Check sheet for the modelled part. Datum: model origin and axes. Units: mm. A direction names the side the tool comes from. Round coordinates to 2 decimals unless told otherwise and drop trailing zeros. Order: outer loops, then holes, each group sorted by start corner. A loop starts at its lowest first (then second) coordinate and runs counter-clockwise, first axis right, second up.
Q1. Cross-section at C-C on x = 13. Record the cut outline in (y, z), then the cut area to 3 significant figures.
Q2. Mould release check, pull along Y, two halves, no side actions. Record for faces 5 (the flat face through (2, -2, 0)), 6 (the flat face through (-4, 0, 0)), 7 (the cylindrical face through (13.68, 4.08, -5.65)), 8 (the cylindrical face through (11.631, 5.175, -4.771)): +Y half, -Y half, draft (parallel to the pull), parting line (faces both ways), or undercut.
Q3. Cross-section at D-D on z = 5. Record the cut outline in (x, y).
Q4. Scan lines: probe 1 along Z at (x, y) = (0, 3.5); probe 2 along Y at (x, z) = (9.25, -2.4); probe 3 along Z at (x, y) = (10, 9.5). Record each from-to range of solid material in increasing order.
Q5. Depth check by flat-ended pin: P1, Ø4, axis at x = 3.5, z = 0, coming from the +Y side; P2, Ø5, axis at x = 9.25, y = 7, coming from the +Z side; P3, Ø4, axis at x = -3, z = -4, coming from the +Y side; P4, Ø0.5, axis at x = -4.5, z = -0.5, coming from the +Y side. Enter the tip coordinate at first touch or a pass-through.
Q6. Set-up check for faces 1 (the flat face through (-4, -1, 1)), 2 (the flat face through (9, 4, -1)), 3 (the flat face through (8, 5.7, -3.25)), 4 (the flat face through (9, 4, 3.75)): record each of +Z, -Z, +X, -X, +Y, -Y from which the full face is reachable in a straight line by a thin tool's end or side.
Q7. Cross-section at B-B on y = 2.5. Record the cut outline in (x, z), then the cut area to 3 significant figures.
Q8. Cross-section at A-A on y = 7. Give the number of separate pieces and of enclosed holes in the cut face, then the cut area to 3 significant figures.
Autodesk Inventor part; units mm, degrees
ref_plane "YZ Plane" through (0, 0, 0) normal (1, 0, 0) x (0, 1, 0)
ref_plane "XZ Plane" through (0, 0, 0) normal (0, 1, 0) x (-1, 0, 0)
ref_plane "XY Plane" through (0, 0, 0) normal (0, 0, 1) x (1, 0, 0)
sketch "Sketch1" plane through (0, 0, 0) normal (0, 1, 0) x (-1, 0, 0)
  circle A0 centre (0, 0) radius 3.75
  dimension "d0" = 7.5
extrude "Extrusion1" add sketch "Sketch1" along normal blind 15
fillet "Fillet1" radius 2 1 edges at (3.75, 15, 0)
sketch "Sketch2" plane through (0, 0, 0) normal (0, -1, 0) x (1, 0, 0)
  line L0 (14.25, 6.25) -> (-6.25, 6.25)
  line L1 (-6.25, 6.25) -> (-6.25, -6.25)
  line L2 (-6.25, -6.25) -> (14.25, -6.25)
  line L3 (14.25, -6.25) -> (14.25, 6.25)
  point P0 (0, 0)
  dimension "d4" = 12.5
  dimension "d5" = 20.5
  dimension "d6" = 6.25
  dimension "d7" = 6.25
extrude "Extrusion2" add sketch "Sketch2" along normal blind 2
sketch "Sketch3" plane through (0, 0, 0) normal (0, 1, 0) x (1, 0, 0)
  line L0 (14.25, -6.25) -> (-6.25, -6.25)
  line L1 (-6.25, 6.25) -> (14.25, 6.25)
  line L2 (-6.25, -6.25) -> (14.25, -6.25)
  line L3 (14.25, -6.25) -> (14.25, 6.25)
  line L4 (14.25, 6.25) -> (-6.25, 6.25)
  line L5 (-6.25, 6.25) -> (-6.25, -6.25)
  circle A0 centre (0, 0) radius 4.65
  point P0 (-6.25, 6.25)
  dimension "d10" = 9.3
extrude "Extrusion3" add sketch "Sketch3" along normal blind 10
sketch "Sketch4" plane through (14.25, -2, 6.25) normal (1, 0, 0) x (0, 0, -1)
  line L0 (5.25, 0) -> (7.25, 0)
  line L1 (7.25, 0) -> (7.25, 12)
  line L2 (7.25, 12) -> (5.25, 12)
  line L3 (5.25, 12) -> (5.25, 0)
  line L4 (12.5, 0) -> (0, 0)
  line L5 (0, 12) -> (12.5, 12)
  line L6 (0, 12) -> (0, 0)
  point P0 (6.25, 2)
  dimension "d14" = 2
  dimension "d15" = 5.25
extrude "Extrusion4" cut sketch "Sketch4" against normal blind 9.71 contours L3 L2 L1 L0
sketch "Sketch6" plane through (0, 10, 0) normal (0, 1, 0) x (1, 0, 0)
  line L0 (6.25, -6.25) -> (12.25, -6.25)
  line L1 (12.25, -6.25) -> (12.25, -3.75)
  line L2 (12.25, -3.75) -> (6.25, -3.75)
  line L3 (6.25, -3.75) -> (6.25, -6.25)
  line L4 (14.25, -6.25) -> (14.25, -1)
  line L5 (-6.25, -6.25) -> (14.25, -6.25)
  point P0 (0, 0)
  dimension "d18" = 6
  dimension "d19" = 2.5
  dimension "d20" = 2
extrude "Extrusion5" cut sketch "Sketch6" against normal through all
sketch "Sketch7" plane through (14.25, -2, -6.25) normal (0, 0, -1) x (-1, 0, 0)
  circle A0 centre (5, 9) radius 1.6
  line L0 (0, 12) -> (20.5, 12)
  line L1 (0, 12) -> (0, 0)
  point P0 (14.25, 2)
  dimension "d23" = 3.2
  dimension "d24" = 3
  dimension "d25" = 5
extrude "Extrusion6" cut sketch "Sketch7" against normal through all
sketch "Sketch8" plane through (14.25, -2, -6.25) normal (0, 0, -1) x (-1, 0, 0)
  circle A0 centre (5, 9) radius 3
  line L0 (0, 12) -> (20.5, 12)
  line L1 (0, 12) -> (0, 0)
  point P0 (14.25, 2)
  dimension "d28" = 6
  dimension "d29" = 3
  dimension "d30" = 5
extrude "Extrusion7" cut sketch "Sketch8" against normal blind 3
fillet "Fillet2" radius 2 3 edges at (-6.25, 4, -6.25) (14.25, 4, -6.25) (-6.25, 4, 6.25)
sketch "Sketch9" plane through (0, 0, 0) normal (0, 1, 0) x (1, 0, 0)
  arc A0 (-4.5412, -1) -> (-4.5412, 1) centre (0, 0) ccw
  arc A1 (-3.6142, -1) -> (-3.6142, 1) centre (0, 0) ccw
  line L0 (14.25, -1) -> (4.5412, -1)
  line L1 (4.5412, 1) -> (14.25, 1)
  line L2 (-4.5412, -1) -> (-3.6142, -1)
  line L3 (-3.6142, 1) -> (-4.5412, 1)
  dimension "d34" = 3.75
  dimension "d35" = 4.65
  dimension "d36" = 2
  dimension "d37" = 2
  dimension "d38" = 2
  dimension "d39" = 2
extrude "Extrusion8" cut sketch "Sketch9" against normal through all
properties part number "BOUCHON"
Results found:
1. outline: (-2, -6.1) - (10, -6.1) - (10, -1) - (-2, -1) - close; (-2, 1) - (10, 1) - (10, 6.25) - (-2, 6.25) - close
1. area: 124 mm2
2. face 5: -Y half
2. face 6: +Y half
2. face 7: draft
2. face 8: undercut
3. outline: (-6.1, -2) - (6.25, -2) - (6.25, 10) - (-6.1, 10) - close; (12.25, -2) - (14.25, -2) - (14.25, 10) - (12.25, 10) - close
4. probe 1: z = -6.25 to -4.65, -3.75 to 3.75, 4.65 to 6.25
4. probe 2: y = -2 to 5.4, 8.6 to 10
4. probe 3: z = -3.25 to -1, 1 to 3.75
5. P1: stops at y = 15
5. P2: stops at z = 3.75
5. P3: stops at y = 14.56
5. P4: stops at y = 10
6. face 1: +Y, -Y
6. face 2: +X, +Y, -Y
6. face 3: -Z
6. face 4: +Z, +Y, -Y
7. outline: (-6.25, -4.25) arc R2 ccw to (-4.25, -6.25) - (12.25, -6.25) arc R2 ccw to (14.25, -4.25) - (14.25, -1) - (4.54, -1) arc R4.65 cw (long way) to (4.54, 1) - (14.25, 1) - (14.25, 6.25) - (12.25, 6.25) - (12.25, 3.75) - (6.25, 3.75) - (6.25, 6.25) - (-4.25, 6.25) arc R2 ccw to (-6.25, 4.25) - close; circle Ø7.5 at (0, 0)
7. area: 196 mm2
8. separate pieces: 4
8. enclosed holes: 0
8. area: 162 mm2
